The listing builds one solid part. Answer for the finished solid, in the listing's coordinates (mm). Coordinates: 2 decimals unless noted, no trailing zeros. Loops run counter-clockwise (first coordinate to the right, second up) from the corner with the lowest first, then second, coordinate; pieces in that order, holes last. Notation, with made-up numbers: (22.5, -1.5) - (58.5, -1.5) arc R22 cw to (58.5, 20.5) - close; hole circle Ø2 at (-1.75, 55). An arc over 180 degrees is marked (long way). Return JSON: item names as keys, results as strings. Group by question number.
1. Each of these flat-tipped pins is pushed along its axis until it touches: P1, Ø3, axis at x = -16.5, y = 28.58, coming from the -Z side; P2, Ø1, axis at y = -47.5, z = 1.5, coming from the -X side. Where does it stop, or does it pass through?
2. Section B-B (y = -7) is taken. Write down the section's boundary in (x, z).
3. Find the intervals of material crossed by line 1 along X through (y, z) = (36, 2.8); line 2 along Y through (x, z) = (22, 0.15); line 3 along Y through (x, z) = (48.5, 1.9), in increasing order.
4. Section C-C (y = 48.5) is taken. Write down the section's boundary in (x, z).
5. Section A-A (x = 0) is taken. Write down the section's boundary in (y, z), and give its area (3 significant figures).
Autodesk Inventor part; units mm, degrees
ref_plane "YZ Plane" through (0, 0, 0) normal (1, 0, 0) x (0, 1, 0)
ref_plane "XZ Plane" through (0, 0, 0) normal (0, 1, 0) x (-1, 0, 0)
ref_plane "XY Plane" through (0, 0, 0) normal (0, 0, 1) x (1, 0, 0)
sketch "Sketch1" plane through (0, 0, 0) normal (0, 0, 1) x (1, 0, 0)
  circle A0 centre (0, 0) radius 29
  circle A1 centre (0, 0) radius 60.5
  line L0 (-40.5, 60.5) -> (40.5, 60.5)
  line L1 (60.5, 40.5) -> (60.5, -40.5)
  line L2 (40.5, -60.5) -> (-40.5, -60.5)
  line L3 (-60.5, -40.5) -> (-60.5, 40.5)
  arc A2 (-40.5, 60.5) -> (-60.5, 40.5) centre (-40.5, 40.5) ccw
  arc A3 (60.5, 40.5) -> (40.5, 60.5) centre (40.5, 40.5) ccw
  arc A4 (40.5, -60.5) -> (60.5, -40.5) centre (40.5, -40.5) ccw
  arc A5 (-60.5, -40.5) -> (-40.5, -60.5) centre (-40.5, -40.5) ccw
  dimension "d0" = 58
  dimension "d1" = 121
  dimension "d2" = 20
extrude "Extrusion1" add sketch "Sketch1" along normal blind 3.18
sketch "Sketch4" plane through (0, 0, 3.18) normal (0, 0, 1) x (1, 0, 0)
  circle A0 centre (0, 0) radius 51.5771
  circle A1 centre (0, 0) radius 43.9861
  circle A2 centre (0, 0) radius 55.7776
  circle A3 centre (0, 0) radius 47.0962
  circle A4 centre (0, 0) radius 42.5777
  circle A5 centre (0, 0) radius 45.3862
  line L0 (0, 0) -> (8.4363, 58.2297)
  line L1 (0, 0) -> (-12.4381, 59.4602)
  line L2 (0, 0) -> (20.1214, 56.5368)
  line L3 (0, 0) -> (38.2622, 45.8865)
  line L4 (0, 0) -> (43.6183, 40.0538)
  line L5 (0, 0) -> (57.1725, 11.9596)
  line L6 (0, 0) -> (57.4745, 1.6902)
  line L7 (0, 0) -> (41.5878, -40.9399)
  line L8 (0, 0) -> (-40.6993, 42.5777)
  line L9 (0, 0) -> (-51.5874, 25.3844)
  line L10 (0, 0) -> (-57.9992, 16.3021)
  line L11 (0, 0) -> (-60.0133, -3.6073)
  line L12 (0, 0) -> (-59.5436, -11.4224)
  line L13 (0, 0) -> (-44.1098, -38.6301)
  line L14 (0, 0) -> (-38.6281, -43.7925)
  line L15 (0, 0) -> (-24.369, -53.7638)
  line L16 (0, 0) -> (-11.9508, -58.1405)
  line L17 (0, 0) -> (5.5489, -59.3314)
  line L18 (0, 0) -> (37.2684, -55.5197)
  line L19 (0, 0) -> (10.7128, -68.7832)
  point P0 (-50.0468, 24.6263)
  point P1 (-42.2573, 20.7934)
  point P2 (-32.5426, 34.0445)
  point P3 (-38.5413, 40.3201)
  point P4 (-55.6771, -3.3466)
  point P5 (-47.0113, -2.8257)
  point P6 (-45.3392, 12.7437)
  point P7 (-53.6968, 15.0928)
  point P8 (-41.9609, -36.7481)
  point P9 (-35.4299, -31.0285)
  point P10 (-46.2528, -8.8728)
  point P11 (-54.7788, -10.5083)
  point P12 (-23.0268, -50.8026)
  point P13 (-19.4428, -42.8955)
  point P14 (-31.1542, -35.3194)
  point P15 (-36.897, -41.83)
  point P16 (5.1939, -55.5352)
  point P17 (4.3855, -46.8915)
  point P18 (-9.4824, -46.1317)
  point P19 (-11.2303, -54.6353)
  point P20 (8.5837, -55.1131)
  point P21 (31.0871, -46.3113)
  point P22 (26.2486, -39.1032)
  point P23 (7.2477, -46.5351)
  point P24 (33.5624, -33.0395)
  point P25 (39.7491, -39.1298)
  point P26 (55.7535, 1.6396)
  point P27 (47.0758, 1.3844)
  point P28 (46.0984, 9.6431)
  point P29 (54.5959, 11.4206)
  point P30 (41.0837, 37.7263)
  point P31 (34.6892, 31.8544)
  point P32 (30.1611, 36.1712)
  point P33 (35.7209, 42.8387)
  point P34 (18.702, 52.5488)
  point P35 (15.7912, 44.3699)
  point P36 (7.9975, 55.2013)
  point P37 (-11.4206, 54.5959)
  point P38 (-9.6431, 46.0984)
  point P39 (6.7528, 46.6095)
  dimension "d76" = 103.1542
  dimension "d78" = 94.1923
extrude "Extrusion4" cut sketch "Sketch4" against normal through all contours A0 L7 A3 L6 | A0 L6 A2 L7 | L5 A3 L4 A0 | A0 L4 A2 L5 | L18 A2 L19 A0 | A0 L19 A3 L18 | L3 A3 L2 A0 | A0 L2 A2 L3 | L17 A2 L16 A0 | A0 L16 A3 L17 | L0 A3 L1 A0 | A0 L1 A2 L0 | L15 A2 L14 A0 | A0 L14 A3 L15 | L8 A3 L9 A0 | A0 L9 A2 L8 | L13 A2 L12 A0 | A0 L12 A3 L13 | L10 A3 L11 A0 | A0 L11 A2 L10
sketch "Sketch5" plane through (0, 0, 3.18) normal (0, 0, 1) x (1, 0, 0)
  circle A0 centre (-48.5, -48.5) radius 2.65
  circle A1 centre (-48.5, 48.5) radius 2.65
  circle A2 centre (48.5, -48.5) radius 2.65
  circle A3 centre (48.5, 48.5) radius 2.65
  circle A4 centre (0, 0) radius 29
  circle A5 centre (0, 0) radius 33
  circle A6 centre (-33, 0) radius 1.25
  circle A7 centre (-16.5, -28.5788) radius 1.25
  circle A8 centre (16.5, -28.5788) radius 1.25
  circle A9 centre (33, 0) radius 1.25
  circle A10 centre (0, 0) radius 65
  line L0 (0, 0) -> (-48.5, -48.5)
  line L1 (0, 0) -> (-46.4652, -66.3592)
  line L2 (0, 0) -> (-57.2887, -40.114)
  circle A11 centre (-37.2825, -53.2449) radius 2.15
  circle A12 centre (-53.2449, -37.2825) radius 2.15
  circle A13 centre (53.2449, -37.2825) radius 2.15
  circle A14 centre (37.2825, -53.2449) radius 2.15
  circle A15 centre (37.2825, 53.2449) radius 2.15
  circle A16 centre (53.2449, 37.2825) radius 2.15
  circle A17 centre (-53.2449, 37.2825) radius 2.15
  circle A18 centre (-37.2825, 53.2449) radius 2.15
  circle A19 centre (16.5, 28.5788) radius 1.25
  circle A20 centre (-16.5, 28.5788) radius 1.25
  dimension "d61" = 66
  dimension "d57" = 5.3
  dimension "d58" = 5.3
  dimension "d59" = 5.3
  dimension "d60" = 5.3
  dimension "d62" = 2.5
  dimension "d65" = 360
  dimension "d67" = 130
  dimension "d68" = 10
  dimension "d69" = 10
  dimension "d70" = 4.3
  dimension "d71" = 4.3
  dimension "d74" = 360
extrude "Extrusion5" cut sketch "Sketch5" against normal through all contours A0 | A12 L2 A10 | A10 L2 A12 | A11 L1 A10 | A10 L1 A11 | L2 A12 A10 | A10 A12 L2 | L1 A11 A10 | A10 A11 L1 | A6 A5 | A5 A6 | A7 A5 | A5 A7 | A17 A10 | A10 A17 | A14 A10 | A10 A14 | A20 A5 | A5 A20 | A8 A5 | A5 A8 | A18 A10 | A10 A18 | A13 A10 | A10 A13 | A19 A5 | A5 A19 | A9 A5 | A5 A9 | A15 A10 | A10 A15 | A16 A10 | A10 A16 | A1 | A2 | A3
sketch "Sketch6" plane through (0, 0, 3.18) normal (0, 0, 1) x (1, 0, 0)
  arc A0 (39.7491, -39.1298) -> (55.7535, 1.6396) centre (0, 0) ccw
  line L0 (64.1152, -33.9991) -> (64.1152, 1.6396)
  line L1 (55.7535, 1.6396) -> (64.1152, 1.6396)
  line L2 (64.1152, -33.9991) -> (46.2085, -31.2396)
  point P0 (47.5954, -29.0829)
  point P1 (55.585, -4.6304)
extrude "Extrusion6" cut sketch "Sketch6" against normal through all
chamfer "Chamfer2" distance 4 angle 45 1 edges at (46.2085, -31.2396, 1.59)
chamfer "Chamfer3" distance 1 angle 45 2 edges at (60.5, 1.6396, 1.59) (60.5, -33.4419, 1.59)
equation "\"d58\" = d57"
equation "\"d59\" = d57"
equation "\"d60\" = d57"
equation "\"d69\" = d68"
properties part number "stator_mount_01_alu"
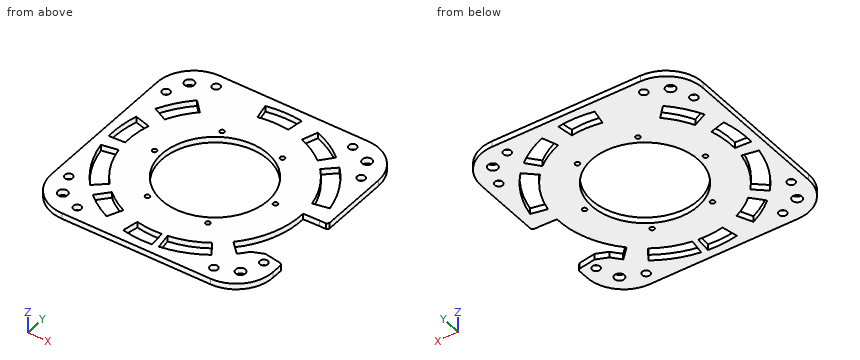
The answers:
{
 "1": {"P1": "stops at z = 0", "P2": "stops at x = -59.41"},
 "2": {"outline": "(-60.5, 0) - (-28.14, 0) - (-28.14, 3.18) - (-60.5, 3.18) - close; (28.14, 0) - (46.57, 0) - (46.57, 3.18) - (28.14, 3.18) - close"},
 "3": {"line 1": "x = -60.5 to -54.97, -51.52 to -42.6, -34.41 to 39.2, 42.6 to 51.52, 54.97 to 60.5", "line 2": "y = -60.5 to -51.26, -41.64 to -18.89, 18.89 to 41.64, 51.26 to 60.5", "line 3": "y = -58.83 to -51.15, -45.85 to -32.54, 1.43 to 10.15, 27.55 to 45.85, 51.15 to 58.83"},
 "4": {"outline": "(-58.83, 0) - (-51.15, 0) - (-51.15, 3.18) - (-58.83, 3.18) - close; (-45.85, 0) - (-10.15, 0) - (-10.15, 3.18) - (-45.85, 3.18) - close; (7.03, 0) - (17.26, 0) - (17.26, 3.18) - (7.03, 3.18) - close; (27.55, 0) - (45.85, 0) - (45.85, 3.18) - (27.55, 3.18) - close; (51.15, 0) - (58.83, 0) - (58.83, 3.18) - (51.15, 3.18) - close"},
 "5": {"outline": "(-60.5, 0) - (-55.78, 0) - (-55.78, 3.18) - (-60.5, 3.18) - close; (-47.1, 0) - (-29, 0) - (-29, 3.18) - (-47.1, 3.18) - close; (29, 0) - (47.1, 0) - (47.1, 3.18) - (29, 3.18) - close; (55.78, 0) - (60.5, 0) - (60.5, 3.18) - (55.78, 3.18) - close", "area": "145 mm2"}
}
